Read the model definition and answer for the solid it produces. Units are mm, in the model's axes. Face numbers are marked on the shaded views. Give positions to 0.01 mm unless a question says otherwise; leave off trailing zeros. Write each loop counter-clockwise with the first axis right and the second up, starting at its lowest first coordinate (ties: lowest second). Pieces come first, ordered by that corner, then holes.
```python
from build123d import *

# Parameters (mm, degrees)
F0_R     = 28.5
F0_R_2   = 1.5
F0_R_3   = 22.5
F1_DEPTH = 3
F2_R     = 1.5
F3_DEPTH = 2


with BuildPart() as f1:
    # F0 (on Top) → F1 (new body)
    with BuildSketch(Plane.XY):
        Circle(F0_R)
        with Locations((-22.5166604984, -13)):
            Circle(F0_R_2, mode=Mode.SUBTRACT)
        with Locations((22.5166604984, -13)):
            Circle(F0_R_2, mode=Mode.SUBTRACT)
        Circle(F0_R_3, mode=Mode.SUBTRACT)
        with Locations((0, 26)):
            Circle(F0_R_2, mode=Mode.SUBTRACT)
    extrude(amount=F1_DEPTH)

    # F2 (on face) → F3 (cut)
    with BuildSketch(Plane.XY.offset(3)):
        with BuildLine():
            ThreePointArc((-1.1991934148, 28.4747596154), (-1.4602599271, 23.6697337179), (2.75, 26))
            ThreePointArc((2.75, 26), (2.3302662821, 27.4602599271), (1.1991934148, 28.4747596154))
            ThreePointArc((1.1991934148, 28.4747596154), (0, 28.5), (-1.1991934148, 28.4747596154))
        make_face()
        with Locations((0, 26)):
            Circle(F2_R, mode=Mode.SUBTRACT)
        with BuildLine():
            ThreePointArc((-19.7666604984, -13), (-22.6161495504, -10.2518002386), (-25.259461901, -13.1988478464))
            ThreePointArc((-25.259461901, -13.1988478464), (-24.6817240079, -14.25), (-24.0602684862, -15.2759117689))
            ThreePointArc((-24.0602684862, -15.2759117689), (-21.2287206641, -15.429755334), (-19.7666604984, -13))
        make_face()
        with Locations((-22.5166604984, -13)):
            Circle(F2_R, mode=Mode.SUBTRACT)
        with BuildLine():
            ThreePointArc((24.0602684862, -15.2759117689), (24.6817240079, -14.25), (25.259461901, -13.1988478464))
            ThreePointArc((25.259461901, -13.1988478464), (25.2648602598, -13.099489052), (25.2666604984, -13))
            ThreePointArc((25.2666604984, -13), (20.0869051644, -11.7120601657), (24.0602684862, -15.2759117689))
        make_face()
        with Locations((22.5166604984, -13)):
            Circle(F2_R, mode=Mode.SUBTRACT)
    extrude(amount=-F3_DEPTH, mode=Mode.SUBTRACT)

    # F4 (on Front) → F5 (revolve, cut)
    with BuildSketch(Plane.XZ):
        Polygon((-23.8397459622, 5), (-22.5, 0), (-22.5, 5), align=None)
    revolve(axis=Axis((0, 0, 2.1961932071), (0, 0, 1)), mode=Mode.SUBTRACT)


solid = f1.part
```
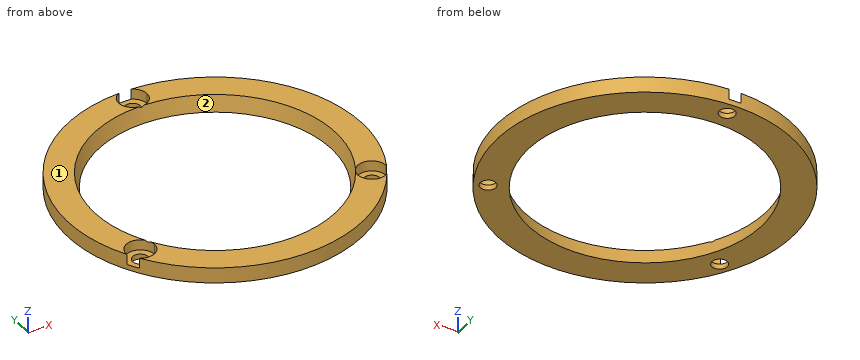
Item 1: Determine the mould class of the marked faces 1 and 2 for opening direction Y: pulls with the +Y half, pulls with the -Y half, needs draft (parallel to the pull), parting line crosses it, or undercut.
Result set:
face 1: needs draft
face 2: undercut
Item 2: Find the intervals of material crossed by line 1 along Y through (x, z) = (20.5, 2.6); line 2 along Y through (x, z) = (-21, 2.3); line 3 along X through (y, z) = (7, 2.55), in increasing order.
Result set:
line 1: y = -19.8 to -14.87, -11.13 to -10.86, 10.86 to 19.8
line 2: y = -19.27 to -15.29, -10.71 to -9.66, 9.66 to 19.27
line 3: x = -27.63 to -22.1, 22.1 to 27.63
Item 3: Each of these flat-tipped pins is pushed along its axis until it touches: pin 1 Ø1 at (x, y) = (20.5, -4.5) entering from +Z; pin 2 Ø2.5 at (x, y) = (0, 26.5) entering from +Z. Where does it stop, or does it pass through?
Result set:
pin 1: passes through
pin 2: stops at z = 1
Item 4: Section B-B (z = 2.4) is taken. Write down the section's boundary in (x, y), and give its area (3 significant figures).
Result set:
outline: (-25.26, -13.2) arc R2.75 cw (long way) to (-24.06, -15.28) arc R28.5 ccw to (24.06, -15.28) arc R2.75 cw (long way) to (25.26, -13.2) arc R28.5 ccw to (1.2, 28.47) arc R2.75 cw (long way) to (-1.2, 28.47) arc R28.5 ccw to start; hole circle Ø46.29 at (0, 0)
area: 799 mm2
Item 5: Section A-A (y = 0) is taken. Write down the section's boundary in (x, z).
Result set:
outline: (-28.5, 0) - (-22.5, 0) - (-23.3, 3) - (-28.5, 3) - close; (22.5, 0) - (28.5, 0) - (28.5, 3) - (23.3, 3) - close
